Autodesk Inventor part; units mm, degrees
ref_plane "YZ Plane" through (0, 0, 0) normal (1, 0, 0) x (0, 1, 0)
ref_plane "XZ Plane" through (0, 0, 0) normal (0, 1, 0) x (-1, 0, 0)
ref_plane "XY Plane" through (0, 0, 0) normal (0, 0, 1) x (1, 0, 0)
sketch "Sketch1" plane through (0, 0, 0) normal (0, 0, 1) x (1, 0, 0)
  circle A0 centre (0, 0) radius 4.25
  circle A1 centre (40, 0) radius 4.25
  circle A2 centre (80, 0) radius 4.25
  circle A3 centre (0, 40) radius 4.25
  circle A4 centre (0, 80) radius 4.25
  line L0 (0, 0) -> (0, 80) construction
  line L1 (0, 0) -> (80, 0) construction
  line L2 (-20, 98) -> (-20, -20)
  line L3 (-20, -20) -> (98, -20)
  line L4 (98, -20) -> (98, 98)
  line L5 (98, 98) -> (-20, 98)
  line L6 (20, 98) -> (98, 20)
  dimension "d0" = 8.5
  dimension "d1" = 8.5
  dimension "d2" = 8.5
  dimension "d3" = 8.5
  dimension "d4" = 8.5
  dimension "d5" = 80
  dimension "d6" = 80
  dimension "d7" = 118
  dimension "d8" = 118
  dimension "d9" = 20
  dimension "d10" = 20
  dimension "d11" = 40
  dimension "d12" = 40
extrude "Extrusion1" add sketch "Sketch1" along normal mid plane 5 contours L5 L6 L4 L3 L2
fillet "Fillet1" radius 3 5 edges at (-20, 98, 0) (20, 98, 0) (-20, -20, 0) (98, 20, 0) (98, -20, 0)
equation "\"d1\" = d0"
equation "\"d2\" = d0"
equation "\"d3\" = d0"
equation "\"d4\" = d0"
equation "\"d6\" = d5"
properties part number "Connection_plate_L_120x120" material "Aluminum 6061"
Verification items for the finished model (mm, model axes). Give positions to 0.01 mm unless a question says otherwise; leave off trailing zeros. Order: outer loops, then holes, each group sorted by start corner. A loop starts at its lowest first (then second) coordinate and runs counter-clockwise, first axis right, second up. Notation, with made-up numbers: M 84.25,37 L 128.25,37 A37 ccw 128.25,75 Z; hole C -0.75,51.5 d7. An arc over 180 degrees is marked long. Answer as a JSON object with one key per item and string values. Group by question number.
1) Cross-section at A-A (y = 80). Enter the section's corners in (x, z).
2) Scan lines: line 1 along Y through (x, z) = (0, -0.2); line 2 along Y through (x, z) = (23, 1.2); line 3 along X through (y, z) = (-1, -0.35). Record each from-to range of solid material in increasing order. Write a range as [from, to].
3) Cross-section at D-D (x = 30). Enter the section's corners in (y, z).
4) Mould release check, pull along Y, two halves, no side actions. Record for faces 1 (the face through (97.14, -19.1, -0.04)), 2 (the face through (35.754, -0.187, -0.035)), 3 (the face through (-20, 40, 0)): released by +Y, released by -Y, zero draft, split by the parting line, or undercut.
5) Depth check by flat-ended pin: pin 1 Ø11 at (x, y) = (0, 80) entering from -Z. Enter the tip coordinate at first touch or a pass-through.
6) Cross-section at C-C (z = -1.4). Enter the section's corners in (x, y).
Result sheet:
{
 "1": {"outline": "M -20,-2.5 L -4.25,-2.5 L -4.25,2.5 L -20,2.5 Z; M 4.25,-2.5 L 38,-2.5 L 38,2.5 L 4.25,2.5 Z"},
 "2": {"line 1": "y = [-20, -4.25], [4.25, 35.75], [44.25, 75.75], [84.25, 98]", "line 2": "y = [-20, 95]", "line 3": "x = [-20, -4.13], [4.13, 35.87], [44.13, 75.87], [84.13, 98]"},
 "3": {"outline": "M -20,-2.5 L 88,-2.5 L 88,2.5 L -20,2.5 Z"},
 "4": {"face 1": "released by -Y", "face 2": "undercut", "face 3": "zero draft"},
 "5": {"pin 1": "stops at z = -2.5"},
 "6": {"outline": "M -20,-17 A3 ccw -17,-20 L 95,-20 A3 ccw 98,-17 L 98,18.76 A3 ccw 97.12,20.88 L 20.88,97.12 A3 ccw 18.76,98 L -17,98 A3 ccw -20,95 Z; hole C 0,0 d8.5; hole C 0,40 d8.5; hole C 0,80 d8.5; hole C 40,0 d8.5; hole C 80,0 d8.5"}
}
